from build123d import *

# Parameters (mm, degrees)
F1_DEPTH  = 0.5
F4_DEPTH  = 1.5
F5_W      = 17.9758077912
F5_H      = 21.7117034923
F5_W_2    = 14.8
F5_H_2    = 6.5
F6_DEPTH  = 0.5
F7_W      = 21
F7_H      = 0.5
F8_DEPTH  = 5
F10_DEPTH = 5
F11_DEPTH = 0.5
F12_DEPTH = 0.5


# Not quite as in the source:
# - a feature names something its author has since deleted; it is built from what else it names


with BuildPart() as f1:
    # F0 (on Top) → F1 (new body)
    with BuildSketch(Plane.XY):
        with BuildLine():
            Line((43.5, 0), (6.5, 0))
            ThreePointArc((6.5, 0), (1.9038059223, -1.9038059223), (0, -6.5))
            Line((0, -6.5), (0, -43.5))
            ThreePointArc((0, -43.5), (1.9038059223, -48.0961940777), (6.5, -50))
            Line((6.5, -50), (43.5, -50))
            ThreePointArc((43.5, -50), (48.0961940777, -48.0961940777), (50, -43.5))
            Line((50, -43.5), (50, -6.5))
            ThreePointArc((50, -6.5), (48.0961940777, -1.9038059223), (43.5, 0))
        make_face()
    extrude(amount=F1_DEPTH)

    # F2 (on face) → F4 (join)
    with BuildSketch(Plane.XY.offset(0.5)):
        with BuildLine():
            Line((43.75, -1.75), (6.25, -1.75))
            ThreePointArc((6.25, -1.75), (2.7144660941, -3.2144660941), (1.25, -6.75))
            Line((1.25, -6.75), (1.25, -43.25))
            ThreePointArc((1.25, -43.25), (2.7144660941, -46.7855339059), (6.25, -48.25))
            Line((6.25, -48.25), (43.75, -48.25))
            ThreePointArc((43.75, -48.25), (47.2855339059, -46.7855339059), (48.75, -43.25))
            Line((48.75, -43.25), (48.75, -6.75))
            ThreePointArc((48.75, -6.75), (47.2855339059, -3.2144660941), (43.75, -1.75))
        make_face()
        with BuildLine():
            ThreePointArc((2.25, -7.75), (3.7144660941, -4.2144660941), (7.25, -2.75))
            Line((7.25, -2.75), (42.75, -2.75))
            ThreePointArc((42.75, -2.75), (46.2855339059, -4.2144660941), (47.75, -7.75))
            Line((47.75, -7.75), (47.75, -42.25))
            ThreePointArc((47.75, -42.25), (46.2855339059, -45.7855339059), (42.75, -47.25))
            Line((42.75, -47.25), (7.25, -47.25))
            ThreePointArc((7.25, -47.25), (3.7144660941, -45.7855339059), (2.25, -42.25))
            Line((2.25, -42.25), (2.25, -7.75))
        make_face(mode=Mode.SUBTRACT)
    extrude(amount=F4_DEPTH)

    # F5 (on face) → F6 (cut, through all)
    with BuildSketch(Plane(origin=(0, 0, 0), x_dir=(1, 0, 0), z_dir=(0, 0, -1))):
        with Locations((15.3125571672, 35.8414453501)):
            Rectangle(F5_W, F5_H)
        with BuildLine():
            Line((40.2913850072, 45.25), (33.4913850072, 45.25))
            ThreePointArc((33.4913850072, 45.25), (32.784278226, 44.9571067812), (32.4913850072, 44.25))
            Line((32.4913850072, 44.25), (32.4913850072, 43.45))
            Line((32.4913850072, 43.45), (33.2634609292, 41.133772234))
            ThreePointArc((33.2634609292, 41.133772234), (33.6274339426, 40.6387578148), (34.2121442272, 40.45))
            Line((34.2121442272, 40.45), (39.5706257871, 40.45))
            ThreePointArc((39.5706257871, 40.45), (40.1553360718, 40.6387578148), (40.5193090852, 41.133772234))
            Line((40.5193090852, 41.133772234), (41.2913850072, 43.45))
            Line((41.2913850072, 43.45), (41.2913850072, 44.25))
            ThreePointArc((41.2913850072, 44.25), (40.9984917884, 44.9571067812), (40.2913850072, 45.25))
        make_face()
        with Locations((37.5, 34.2)):
            Rectangle(F5_W_2, F5_H_2)
    extrude(amount=-F6_DEPTH, mode=Mode.SUBTRACT)

    # F7 (on face) → F8 (join)
    with BuildSketch(Plane.XY.offset(0.5)):
        with Locations((37.25, -39.1)):
            Rectangle(F7_W, F7_H)
        Polygon((37.75, -26.95), (47.75, -26.95), (47.75, -26.45), (27.75, -26.45), (27.75, -26.95), align=None)
    extrude(amount=F8_DEPTH)

    # F9 (on face) → F10 (join)
    with BuildSketch(Plane.XY.offset(0.5)):
        Polygon((46.7340297326, -11.4003978506), (46.7340297326, -15.1797328308), (47.2340297326, -15.2791890145), (47.2340297326, -11.3009416669), align=None)
        Polygon((39.1236972228, -22.7900653407), (35.3443622425, -22.7900653407), (35.2449060588, -23.2900653407), (39.2231534064, -23.2900653407), align=None)
        Polygon((27.2340297326, -15.2791890145), (27.7340297326, -15.1797328308), (27.7340297326, -11.4003978506), (27.2340297326, -11.3009416669), align=None)
        Polygon((17.1048343345, -22.7900653407), (17.0053781508, -22.2900653407), (13.424955538, -22.2900653407), (13.3254993543, -22.7900653407), align=None)
        Polygon((24.2151668444, -11.4998540343), (24.2151668444, -15.0802766471), (24.7151668444, -15.1797328308), (24.7151668444, -11.4003978506), align=None)
        Polygon((5.7151668444, -15.1797328308), (6.2151668444, -15.0802766471), (6.2151668444, -11.4998540343), (5.7151668444, -11.4003978506), align=None)
    extrude(amount=F10_DEPTH)

    # F9 (on face) → F11 (cut, through all)
    with BuildSketch(Plane.XY.offset(0.5)):
        Polygon((27.7340297326, -15.1797328308), (29.1803186149, -18.6713830655), (31.8527120078, -21.3437764584), (35.3443622425, -22.7900653407), (39.1236972228, -22.7900653407), (42.6153474575, -21.3437764584), (45.2877408504, -18.6713830655), (46.7340297326, -15.1797328308), (46.7340297326, -11.4003978506), (45.2877408504, -7.9087476159), (42.6153474575, -5.236354223), (39.1236972228, -3.7900653407), (35.3443622425, -3.7900653407), (31.8527120078, -5.236354223), (29.1803186149, -7.9087476159), (27.7340297326, -11.4003978506), align=None)
    extrude(amount=-F11_DEPTH, mode=Mode.SUBTRACT)

    # F9 (on face) → F12 (cut, through all)
    with BuildSketch(Plane.XY.offset(0.5)):
        Polygon((22.8449984296, -18.3881558169), (24.2151668444, -15.0802766471), (24.2151668444, -11.4998540343), (22.8449984296, -8.1919748645), (20.3132573206, -5.6602337555), (17.0053781508, -4.2900653407), (13.424955538, -4.2900653407), (10.1170763683, -5.6602337555), (7.5853352592, -8.1919748645), (6.2151668444, -11.4998540343), (6.2151668444, -15.0802766471), (7.5853352592, -18.3881558169), (10.1170763683, -20.9198969259), (13.424955538, -22.2900653407), (17.0053781508, -22.2900653407), (20.3132573206, -20.9198969259), align=None)
    extrude(amount=-F12_DEPTH, mode=Mode.SUBTRACT)


solid = f1.part
Here's how the part is built. I have some questions about the finished solid (model axes, mm). A direction names the side the tool comes from. Give positions to 0.01 mm unless a question says otherwise; leave off trailing zeros. Order: outer loops, then holes, each group sorted by start corner. A loop starts at its lowest first (then second) coordinate and runs counter-clockwise, first axis right, second up. Notation, with made-up numbers: (45.25, 63.5) -> (53.25, 63.5) arc R31 cw to (53.25, 89.5) -> close; hole circle Ø7 at (-29.5, 62.5). An arc over 180 degrees is marked (long way). Use a Markdown table: item, result. Add a question column.
Item 1: I need wall thicknesses on line 1 (X direction, y = -12, z = 2.5); line 2 (Y direction, x = 16.5, z = 0.85); line 3 (Y direction, x = 40, z = 4.35). Which ranges of each line are inside material? Lowest first, please.
Item 2: Imagine slicing it at B-B on x = 14.5. Please give me the cut outline in (y, z), plus the area to 3 significant figures.
Item 3: Imagine slicing it at D-D on y = -12.5. Please give me the cut outline in (x, z), plus the area to 3 significant figures.
Item 4: Imagine slicing it at C-C on z = 1.35. Give the number of separate pieces and of enclosed holes in the cut face, plus the area to 3 significant figures.
Item 5: Imagine slicing it at A-A on y = -34. Please give me the cut outline in (x, z), plus the area to 3 significant figures.
Item 6: If we mould it in two halves opening along Y, with no side actions, what happens to faces 5 (the face through (2.68, -46.75, 1.24)), 6 (the face through (25, -25, 0.5)), 7 (the face through (48.146, -1.955, 0.246))? For each: pulls with the +Y half, pulls with the -Y half, needs draft (parallel to the pull), parting line crosses it, or undercut.
Item 7: Will these pins go through, and if not, where does the flat tip stop? pin 1 (1.1 mm diameter, centred on y = -14, z = 4, fed in from +X); pin 2 (15 mm diameter, centred on x = 19, y = -14, fed in from +Z); pin 3 (8 mm diameter, centred on x = 34.5, y = -14.5, fed in from -Z) (3 decimals); pin 4 (1.2 mm diameter, centred on y = -13, z = 2, fed in from -X).
Item 8: For faces 1 (the face through (1.854, -48.045, 0.246)), 2 (the face through (23.52, -16.76, 0.25)), 3 (the face through (25, -48.25, 1)), 4 (the face through (2.25, -25, 1)), which set-ups out of +Z, -Z, +X, -X, +Y, -Y let a thin tool reach every point of the face, with its end or its side?
Data:
| question | item | result |
|---|---|---|
| 1 | line 1 | x = 5.72 to 6.22, 24.22 to 24.72, 27.23 to 27.73, 46.73 to 47.23 |
| 1 | line 2 | y = -48.25 to -47.25, -22.79 to -22.29, -2.75 to -1.75 |
| 1 | line 3 | y = -39.35 to -38.85, -26.95 to -26.45 |
| 2 | outline | (-50, 0) -> (-46.7, 0) -> (-46.7, 0.5) -> (-47.25, 0.5) -> (-47.25, 2) -> (-48.25, 2) -> (-48.25, 0.5) -> (-50, 0.5) -> close; (-24.99, 0) -> (-22.29, 0) -> (-22.29, 5.5) -> (-22.79, 5.5) -> (-22.79, 0.5) -> (-24.99, 0.5) -> close; (-4.29, 0) -> (0, 0) -> (0, 0.5) -> (-1.75, 0.5) -> (-1.75, 2) -> (-2.75, 2) -> (-2.75, 0.5) -> (-4.29, 0.5) -> close |
| 2 | area | 10.6 mm² |
| 3 | outline | (0, 0) -> (6.22, 0) -> (6.22, 5.5) -> (5.72, 5.5) -> (5.72, 0.5) -> (2.25, 0.5) -> (2.25, 2) -> (1.25, 2) -> (1.25, 0.5) -> (0, 0.5) -> close; (24.22, 0) -> (27.73, 0) -> (27.73, 5.5) -> (27.23, 5.5) -> (27.23, 0.5) -> (24.72, 0.5) -> (24.72, 5.5) -> (24.22, 5.5) -> close; (46.73, 0) -> (50, 0) -> (50, 0.5) -> (48.75, 0.5) -> (48.75, 2) -> (47.75, 2) -> (47.75, 0.5) -> (47.23, 0.5) -> (47.23, 5.5) -> (46.73, 5.5) -> close |
| 3 | area | 19.5 mm² |
| 4 | separate pieces | 7 |
| 4 | enclosed holes | 1 |
| 4 | area | 216 mm² |
| 5 | outline | (0, 0) -> (6.32, 0) -> (6.32, 0.5) -> (2.25, 0.5) -> (2.25, 2) -> (1.25, 2) -> (1.25, 0.5) -> (0, 0.5) -> close; (24.3, 0) -> (30.1, 0) -> (30.1, 0.5) -> (24.3, 0.5) -> close; (44.9, 0) -> (50, 0) -> (50, 0.5) -> (48.75, 0.5) -> (48.75, 2) -> (47.75, 2) -> (47.75, 0.5) -> (44.9, 0.5) -> close |
| 5 | area | 11.6 mm² |
| 6 | face 5 | pulls with the -Y half |
| 6 | face 6 | undercut |
| 6 | face 7 | pulls with the +Y half |
| 7 | pin 1 | stops at x = 47.23 |
| 7 | pin 2 | stops at z = 5.5 |
| 7 | pin 3 | passes through |
| 7 | pin 4 | stops at x = 1.25 |
| 8 | face 1 | +Z, -Z, -X, -Y |
| 8 | face 2 | +Z, -Z |
| 8 | face 3 | +Z, +X, -X, -Y |
| 8 | face 4 | +Z |
